```python
from build123d import *

# Parameters (mm, degrees)
SKETCH1_W           = 304.8
SKETCH1_H           = 210
BOSS_EXTRUDE1_DEPTH = 12.7
SKETCH2_W           = 103.826139809
SKETCH2_H           = 75.404069631
SKETCH2_W_2         = 105.873975136
CUT_EXTRUDE1_DEPTH  = 121


with BuildPart() as part:
    # Sketch1 → Boss-Extrude1 (new body)
    with BuildSketch(Plane(origin=(0, 0, 0), x_dir=(1, 0, 0), z_dir=(0, 1, 0))):
        Rectangle(SKETCH1_W, SKETCH1_H)
    extrude(amount=BOSS_EXTRUDE1_DEPTH)

    # Sketch2 → Cut-Extrude1 (cut)
    with BuildSketch(Plane.XZ):
        with Locations((-115.413069905, -104.602034816)):
            Rectangle(SKETCH2_W, SKETCH2_H)
        with Locations((127.97392141, -104.602034816)):
            Rectangle(SKETCH2_W_2, SKETCH2_H)
    extrude(amount=-CUT_EXTRUDE1_DEPTH, mode=Mode.SUBTRACT)


solid = part.part
```
Source: CAD feature listing. Evaluate the final solid. Frame: model axes, mm. A direction names the side the tool comes from. Coordinates: 2 decimals unless noted, no trailing zeros. Write each loop counter-clockwise with the first axis right and the second up, starting at its lowest first coordinate (ties: lowest second). Pieces come first, ordered by that corner, then holes. Notation, with made-up numbers: (40, 52) -> (73, 52) arc R25 cw to (73, 70) -> close; hole circle Ø10 at (-39.75, 38). An arc over 180 degrees is marked (long way). Return JSON: item names as keys, results as strings. Group by question number.
1) Contact query for flat-ended pins moving along their axis: P1, Ø2, axis at y = 11, z = -80.5, coming from the +X side; P2, Ø6.5, axis at x = -93, y = 7, coming from the -Z side. Output: stop coordinate, or through.
2) Section query A-A, the plane y = 3. Return loops of the section in (x, z), plus the area to 3 significant figures.
3) Ray query, line 1 along Z through (x, y) = (-105, 1.5); line 2 along X through (y, z) = (4, -71.5). Return the intervals inside material, ascending.
4) Set-up query: faces 1 (the face through (-152.4, 6, 20)), 2 (the face through (-63.5, 6, -86)), 3 (the face through (113, 6, -66.9)). Return all of +Z, -Z, +X, -X, +Y, -Y with unobstructed straight access to the full face (end or side cutting, diameter ignored); none if empty.
5) Section query B-B, the plane x = -73.5. Return loops of the section in (y, z).
From the geometry:
{
 "1": {"P1": "x = 75.04", "P2": "z = -66.9"},
 "2": {"outline": "(-152.4, -66.9) -> (-63.5, -66.9) -> (-63.5, -105) -> (75.04, -105) -> (75.04, -66.9) -> (152.4, -66.9) -> (152.4, 105) -> (-152.4, 105) -> close", "area": "57,700 mm²"},
 "3": {"line 1": "-66.9 to 105", "line 2": "-63.5 to 75.04"},
 "4": {"face 1": "+Z, -Z, -X, +Y, -Y", "face 2": "-Z, -X, +Y, -Y", "face 3": "-Z, +X, +Y, -Y"},
 "5": {"outline": "(0, -66.9) -> (12.7, -66.9) -> (12.7, 105) -> (0, 105) -> close"}
}
